from build123d import *

# Parameters (mm, degrees)
MODEL_R                         = 1.6
AUFSATZ_LINEAR_AUSTRAGEN1_DEPTH = 2


with BuildPart() as part:
    # Model → Aufsatz-Linear austragen1 (new body)
    with BuildSketch(Plane.XY):
        with BuildLine():
            Line((60, 0), (60, 49))
            ThreePointArc((60, 49), (18.375108617, 38.734560877), (0, 0))
            Line((0, 0), (60, 0))
        make_face()
        with Locations((20, 5)):
            Circle(MODEL_R, mode=Mode.SUBTRACT)
        with Locations((55, 30)):
            Circle(MODEL_R, mode=Mode.SUBTRACT)
        with Locations((55, 5)):
            Circle(MODEL_R, mode=Mode.SUBTRACT)
    extrude(amount=AUFSATZ_LINEAR_AUSTRAGEN1_DEPTH)


solid = part.part
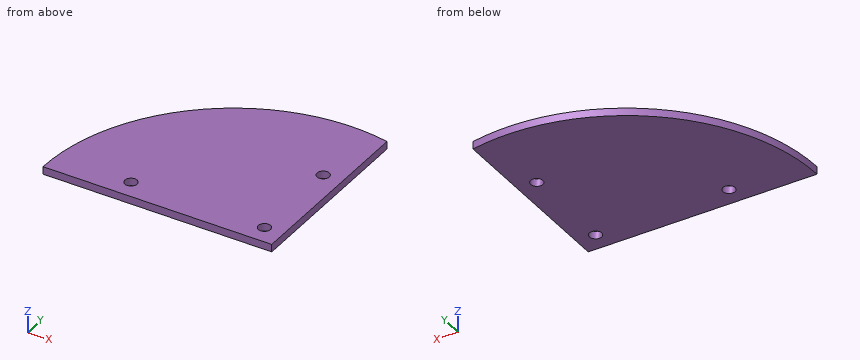
Geometry check sheet. Reference: the model listing, model coordinates, mm. Round coordinates to 2 decimals unless told otherwise and drop trailing zeros. Order: outer loops, then holes, each group sorted by start corner. A loop starts at its lowest first (then second) coordinate and runs counter-clockwise, first axis right, second up. Notation, with made-up numbers: M 5.5,15 L 49.5,15 A12 cw 49.5,27 Z; hole C -29.5,55 d5. An arc over 180 degrees is marked long. Write each question's results on one line, items separated by ' | '. Start each with the question number.
1. Cross-section at D-D on x = 20. Record the boundary of the cut face in (y, z).
2. Go/stop test with a flat-tipped pin: P1, Ø2.5, axis at x = 55, y = 5, coming from the -Z side. Record where the tip stops, or that it passes through.
3. Cross-section at C-C on y = 30. Record the boundary of the cut face in (x, z).
4. Cross-section at B-B on x = 55. Record the boundary of the cut face in (y, z), plus the area to 3 significant figures.
5. Material ranges on L1, parallel to X at y = 4.5, z = 1.75; L2, parallel to Y at x = 55, z = 1.3; L3, parallel to Y at x = 20, z = 1.3, recorded low to high. Write a range as from..to.
6. Cross-section at A-A on z = 0.95. Record the boundary of the cut face in (x, y) (3 decimals), plus the area to 3 significant figures.
Resolved:
1) outline: M 0,0 L 3.4,0 L 3.4,2 L 0,2 Z; M 6.6,0 L 40.01,0 L 40.01,2 L 6.6,2 Z
2) P1: through
3) outline: M 10,0 L 53.4,0 L 53.4,2 L 10,2 Z; M 56.6,0 L 60,0 L 60,2 L 56.6,2 Z
4) outline: M 0,0 L 3.4,0 L 3.4,2 L 0,2 Z; M 6.6,0 L 28.4,0 L 28.4,2 L 6.6,2 Z; M 31.6,0 L 49.76,0 L 49.76,2 L 31.6,2 Z | area: 86.7 mm2
5) L1: 0.2..18.48, 21.52..53.48, 56.52..60 | L2: 0..3.4, 6.6..28.4, 31.6..49.76 | L3: 0..3.4, 6.6..40.01
6) outline: M 0,0 L 60,0 L 60,49 A50.005 ccw Z; hole C 20,5 d3.2; hole C 55,5 d3.2; hole C 55,30 d3.2 | area: 2,440 mm2
